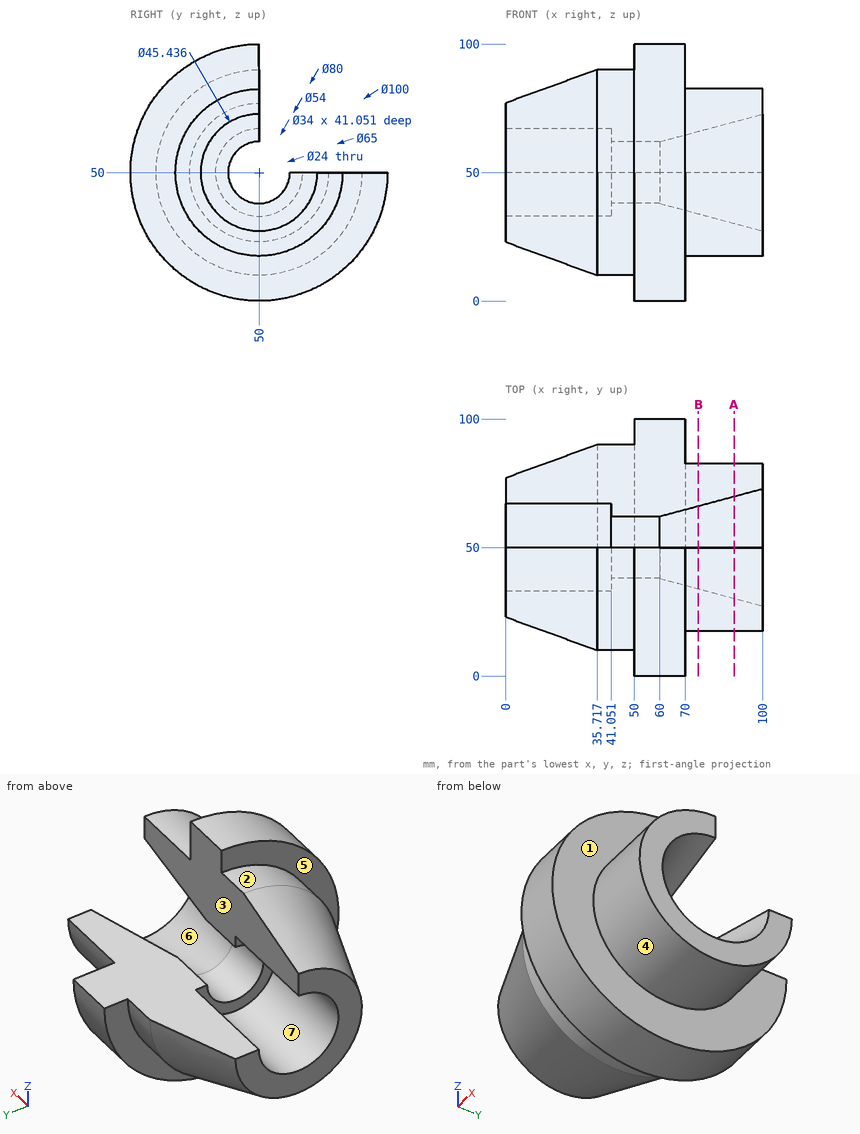
Print and shaded views of the part. All mm, measured from the part's lowest x, y and z. A direction names the side the tool comes from. Round coordinates to 2 decimals unless told otherwise and drop trailing zeros. Write each loop counter-clockwise with the first axis right and the second up, starting at its lowest first coordinate (ties: lowest second). Pieces come first, ordered by that corner, then holes.
(1) Slice it at A-A, the plane x = 89. Write the cut outline in (y, z), and give its area (3 significant figures).
(2) Drop flat-ended pins along their axis: P1, Ø21.5, axis at y = 50, z = 50, coming from the +X side; P2, Ø4, axis at y = 35, z = 66.5, coming from the +X side; P3, Ø10, axis at y = 44, z = 58, coming from the -X side; P4, Ø10, axis at x = 14, z = 51, coming from the -Y side (1 decimal). Give the stop position or say it passes through.
(3) Mould opens along Y. For the marked faces 4, 5, 6 and 7 say: pulls with the +Y half, pulls with the -Y half, needs draft (parallel to the pull), parting line crosses it, or undercut.
(4) 3-axis set-ups, long thin cutter, end or side, ignore diameter. For the marked faces 1, 2 and 3: which of +Z, -Z, +X, -X, +Y, -Y reach the whole face in a straight line?
(5) Probe line 1 along Z through (x, y) = (29, 21.5); line 2 along Y through (x, z) = (29, 45); line 3 along Z through (x, y) = (51, 70.5) (1 decimal). List the from-to ranges inside material, lowest first.
(6) Slice it at B-B, the plane x = 75. Write the cut outline in (y, z).
From the geometry:
1. outline: (50, 69.77) - (50, 82.5) arc R32.5 ccw (long way) to (82.5, 50) - (69.77, 50) arc R19.77 cw (long way) to start
1. area: 1,570 mm2
2. P1: passes through
2. P2: stops at x = 100
2. P3: stops at x = 41.05
2. P4: stops at y = 16.1
3. face 4: parting line crosses it
3. face 5: needs draft
3. face 6: undercut
3. face 7: undercut
4. face 1: +X
4. face 2: -X
4. face 3: +Z, +X, -X, +Y
5. line 1: z = 25.54 to 74.46
5. line 2: y = 12.78 to 33.75, 66.25 to 87.22
5. line 3: z = 4.4 to 50
6. outline: (50, 66.02) - (50, 82.5) arc R32.5 ccw (long way) to (82.5, 50) - (66.02, 50) arc R16.02 cw (long way) to start
